Job drawing, mm, ordinate dimensions from the low corner. One solid piece. Give positions to 0.01 mm unless a question says otherwise; leave off trailing zeros. Write each loop counter-clockwise with the first axis right and the second up, starting at its lowest first coordinate (ties: lowest second). Pieces come first, ordered by that corner, then holes. Notation, with made-up numbers: (80, -4.5) - (130, -4.5) arc R6 cw to (130, 4.5) - close; hole circle Ø9 at (-21.75, 12.25). An arc over 180 degrees is marked (long way). Use a Markdown table: item, result. Add a question column.
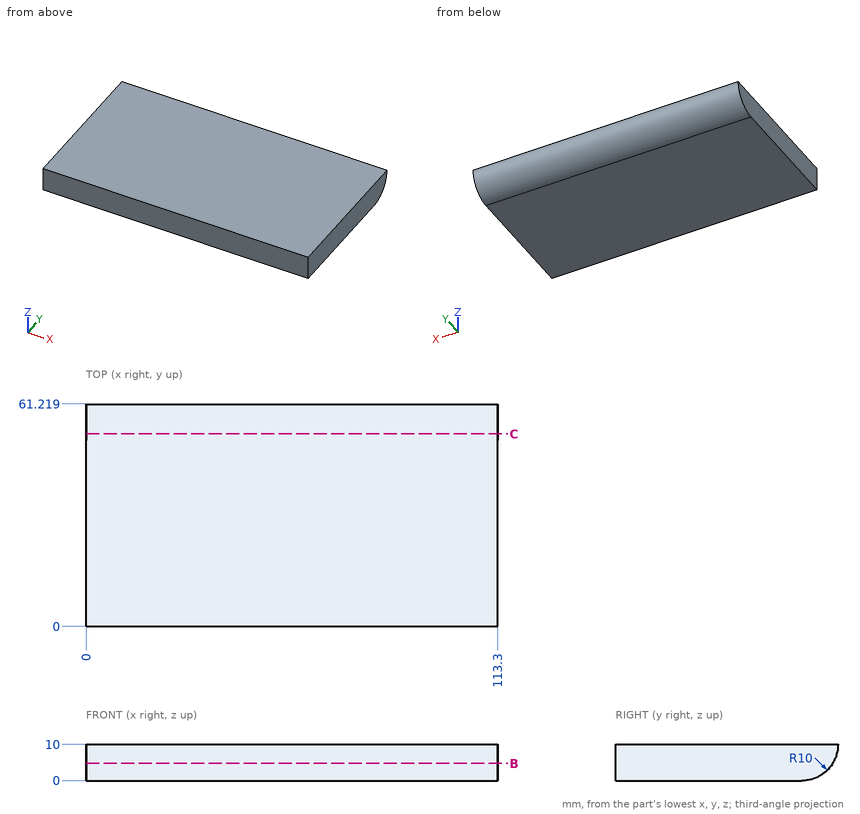
(1) Probe probe 1 along Y at (x, z) = (93, 5); probe 2 along Y at (x, z) = (106, 4); probe 3 along Z at (x, y) = (16.5, 54) (1 decimal). List the from-to ranges inside material, lowest first. Write a range as [from, to].
(2) Band-saw the part on C-C (y = 53). Write the cut outline in (x, z).
(3) Band-saw the part on B-B (z = 4.75). Write the cut outline in (x, y).
(4) Flat gauge pin, fed straight in: pin 1 (1.5 mm diameter, centred on x = 41, z = 9, fed in from +Y) (1 decimal). Where does the tip first touch, or does it go through?
Model answer:
| question | item | result |
|---|---|---|
| 1 | probe 1 | y = [0, 59.88] |
| 1 | probe 2 | y = [0, 59.22] |
| 1 | probe 3 | z = [0.4, 10] |
| 2 | outline | (0, 0.16) - (113.3, 0.16) - (113.3, 10) - (0, 10) - close |
| 3 | outline | (0, 0) - (113.3, 0) - (113.3, 59.73) - (0, 59.73) - close |
| 4 | pin 1 | stops at y = 61.2 |
